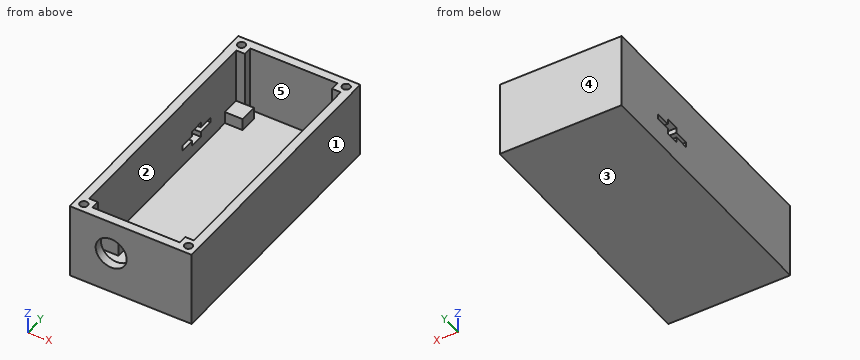
from build123d import *

# Parameters (mm, degrees)
SKETCH_W          = 35.3624
SKETCH_H          = 77.7328
PAD_DEPTH         = 16
PAD_DEPTH_BACK    = 6
SKETCH002_W       = 30.3624
SKETCH002_H       = 72.7328
POCKET_DEPTH      = 3.5
POCKET_DEPTH_BACK = 16
SKETCH003_W       = 5
SKETCH003_H       = 5
PAD001_DEPTH      = 16
PAD001_DEPTH_BACK = 3.5
SKETCH004_W       = 5.1844
SKETCH004_H       = 5.1948
SKETCH004_H_2     = 5
PAD002_DEPTH      = 3.5
SKETCH005_W       = 5.1844
SKETCH005_H       = 2.5
PAD003_DEPTH      = 1.6
PAD003_DEPTH_BACK = 3.5
SKETCH006_R       = 1.15
POCKET001_DEPTH   = 8
SKETCH007_R       = 4.5
POCKET002_DEPTH   = 2.5
POCKET003_DEPTH   = 2.5


with BuildPart() as part:
    # Sketch → Pad (new body, two sides)
    with BuildSketch(Plane.XY) as pad_sk:
        with Locations((14.6812, 25.8664)):
            Rectangle(SKETCH_W, SKETCH_H)
    extrude(amount=PAD_DEPTH)
    extrude(pad_sk.sketch, amount=-PAD_DEPTH_BACK)

    # Sketch002 → Pocket (cut, two sides)
    with BuildSketch(Plane.XY) as pocket_sk:
        with Locations((14.6812, 25.8664)):
            Rectangle(SKETCH002_W, SKETCH002_H)
    extrude(amount=-POCKET_DEPTH, mode=Mode.SUBTRACT)
    extrude(pocket_sk.sketch, amount=POCKET_DEPTH_BACK, mode=Mode.SUBTRACT)

    # Sketch003 → Pad001 (join, two sides)
    with BuildSketch(Plane.XY) as pad001_sk:
        with Locations((29.8624, -10.5)):
            Rectangle(SKETCH003_W, SKETCH003_H)
        with Locations((-0.5, -10.5)):
            Rectangle(SKETCH003_W, SKETCH003_H)
        with Locations((-0.5, 62.2328)):
            Rectangle(SKETCH003_W, SKETCH003_H)
        with Locations((29.8624, 62.2328)):
            Rectangle(SKETCH003_W, SKETCH003_H)
    extrude(amount=PAD001_DEPTH)
    extrude(pad001_sk.sketch, amount=-PAD001_DEPTH_BACK)

    # Sketch004 → Pad002 (join)
    with BuildSketch(Plane.XY):
        with Locations((2.0922, 57.1354)):
            Rectangle(SKETCH004_W, SKETCH004_H)
        with Locations((27.2702, 57.1354)):
            Rectangle(SKETCH004_W, SKETCH004_H)
        with Locations((2.0922, 2.174)):
            Rectangle(SKETCH004_W, SKETCH004_H_2)
        with Locations((27.2702, 2.174)):
            Rectangle(SKETCH004_W, SKETCH004_H_2)
    extrude(amount=-PAD002_DEPTH)

    # Sketch005 → Pad003 (join, two sides)
    with BuildSketch(Plane.XY) as pad003_sk:
        with Locations((27.2702, -1.576)):
            Rectangle(SKETCH005_W, SKETCH005_H)
        with Locations((2.0922, -1.576)):
            Rectangle(SKETCH005_W, SKETCH005_H)
    extrude(amount=PAD003_DEPTH)
    extrude(pad003_sk.sketch, amount=-PAD003_DEPTH_BACK)

    # Sketch006 (on DatumPlane) → Pocket001 (cut)
    with BuildSketch(Plane.XY.offset(16)):
        with Locations((29.8624, -10.5)):
            Circle(SKETCH006_R)
        with Locations((-0.5, -10.5)):
            Circle(SKETCH006_R)
        with Locations((29.8624, 62.2328)):
            Circle(SKETCH006_R)
        with Locations((-0.5, 62.2328)):
            Circle(SKETCH006_R)
    extrude(amount=-POCKET001_DEPTH, mode=Mode.SUBTRACT)

    # Sketch007 (on DatumPlane) → Pocket002 (cut)
    with BuildSketch(Plane.XZ.offset(13)):
        with Locations((9, 6.25)):
            Circle(SKETCH007_R)
    extrude(amount=-POCKET002_DEPTH, mode=Mode.SUBTRACT)

    # Sketch008 (on DatumPlane) → Pocket003 (cut)
    with BuildSketch(Plane(origin=(-3, 0, 0), x_dir=(0, -1, 0), z_dir=(-1, 0, 0))):
        Polygon((-47.9278, 2.85), (-43.4528, 2.85), (-43.4528, 4.35), (-39.4528, 4.35), (-39.4528, 2.85), (-34.9778, 2.85), (-34.9778, 1.35), (-39.4528, 1.35), (-39.4528, -0.15), (-43.4528, -0.15), (-43.4528, 1.35), (-47.9278, 1.35), align=None)
    extrude(amount=-POCKET003_DEPTH, mode=Mode.SUBTRACT)


solid = part.part
The model under review builds one solid part; all positions refer to its coordinate system, in mm. Face numbers are marked on the shaded views. A direction names the side the tool comes from. Give positions to 0.01 mm unless a question says otherwise; leave off trailing zeros. Order: outer loops, then holes, each group sorted by start corner. A loop starts at its lowest first (then second) coordinate and runs counter-clockwise, first axis right, second up. Notation, with made-up numbers: M -37,26 L 9,26 A18 cw 9,57 Z; hole C 58,43.25 d6. An arc over 180 degrees is marked long. Use one line per item in the form item = value. Start each with the question number.
Item 1: We need section C-C on y = 11. Give the boundary of the cut face in (x, z), plus the area to 3 significant figures.
Item 2: The part is to be moulded in two halves that separate along X. For the marked faces 1, 2 and 3, say which applies: pulls with the +X half, pulls with the -X half, needs draft (parallel to the pull), parting line crosses it, or undercut.
Item 3: For the marked faces 4 and 5, list the 3-axis set-ups (+Z, -Z, +X, -X, +Y, -Y) from which the entire face can be reached by the end or side of a thin tool; tool diameter is ignored.
Item 4: We need section A-A on y = 42. Give the boundary of the cut face in (x, z).
Item 5: We need section D-D on x = 19.5. Give the boundary of the cut face in (y, z).
Item 6: To check wall thickness, follow line 1 along Y through (x, z) = (15, 2.5); line 2 along Y through (x, z) = (29.5, 8.5); line 3 along X through (y, z) = (40.5, 5). State the ranges of each line that lie inside material, in increasing order. Write a range as from..to.
Item 7: Insertion check: pin 1 Ø1.1 at (x, y) = (30.5, 61.5) entering from +Z; pin 2 Ø6 at (x, y) = (20.5, 21.5) entering from +Z; pin 3 Ø1.4 at (x, y) = (29.86, -10.5) entering from +Z. Each pin has a flat end and moves straight along its axis. Give the tip position at first contact, or say it passes through.
Item 8: We need section B-B on x = 9. Give the boundary of the cut face in (y, z), plus the area to 3 significant figures.
Completed:
q1.outline = M -3,-6 L 32.36,-6 L 32.36,16 L 29.86,16 L 29.86,-3.5 L -0.5,-3.5 L -0.5,16 L -3,16 Z
q1.area = 186 mm²
q2.face_1 = pulls with the +X half
q2.face_2 = undercut
q2.face_3 = needs draft
q3.face_4 = +Z, -Z, +X, -X, +Y
q3.face_5 = +Z
q4.outline = M -3,-6 L 32.36,-6 L 32.36,16 L 29.86,16 L 29.86,-3.5 L -0.5,-3.5 L -0.5,-0.15 L -3,-0.15 Z; M -3,4.35 L -0.5,4.35 L -0.5,16 L -3,16 Z
q5.outline = M -13,-6 L 64.73,-6 L 64.73,16 L 62.23,16 L 62.23,-3.5 L -10.5,-3.5 L -10.5,16 L -13,16 Z
q6.line_1 = -13..-10.5, 62.23..64.73
q6.line_2 = -13..-11.59, -9.41..-8, 59.73..61.14, 63.32..64.73
q6.line_3 = -3..-0.5, 29.86..32.36
q7.pin_1 = 16
q7.pin_2 = -3.5
q7.pin_3 = 8
q8.outline = M -13,-6 L 64.73,-6 L 64.73,16 L 62.23,16 L 62.23,-3.5 L -10.5,-3.5 L -10.5,1.75 L -13,1.75 Z; M -13,10.75 L -10.5,10.75 L -10.5,16 L -13,16 Z
q8.area = 269 mm²
